from build123d import *

# Parameters (mm, degrees)
F4_D    = 6.4
F5_SIZE = 2


with BuildPart() as f1:
    # F0 (on Front) → F1 (revolve)
    with BuildSketch(Plane.XZ):
        Polygon((-44, 0), (-44, -2), (-2.715, -2), (-2.715, 10), (-60, 10), (-60, 0), align=None)
    revolve(axis=Axis((0, 0, 2.463164), (0, 0, -1)))

    # F4 (through all)
    with Locations(Plane.XY.offset(10)):
        with Locations((-26, 45.033321), (-52, 0), (-26, -45.033321), (26, -45.033321), (52, 0), (26, 45.033321)):
            Hole(F4_D / 2)

    # F5
    f5_edges = [f1.edges().sort_by_distance(p)[0] for p in [
        (60, 0, 10),
    ]]
    chamfer(f5_edges, length=F5_SIZE)

    # F6 (on Front) → F7 (revolve)
    with BuildSketch(Plane.XZ):
        with BuildLine():
            Line((-3.91, 45.97), (-3.91, 37.61))
            Line((-3.91, 37.61), (-5.085, 35.51))
            Line((-5.085, 35.51), (-5.085, 33.81))
            Line((-5.085, 33.81), (-3.91, 33.81))
            Line((-3.91, 33.81), (-3.91, 29.6))
            Line((-3.91, 29.6), (-5.09, 23.4))
            Line((-5.09, 23.4), (-5.09, 20.8))
            Line((-5.09, 20.8), (-3.91, 14.6))
            Line((-3.91, 14.6), (-6.95, 14.6))
            Line((-6.95, 14.6), (-6.95, 10))
            Line((-6.95, 10), (-2.715, 10))
            Line((-2.715, 10), (-2.715, 46.47))
            Line((-2.715, 46.47), (-3.41, 46.47))
            ThreePointArc((-3.41, 46.47), (-3.763553, 46.323553), (-3.91, 45.97))
        make_face()
    revolve(axis=Axis((0, 0, 24.371663), (0, 0, 1)))


solid = f1.part
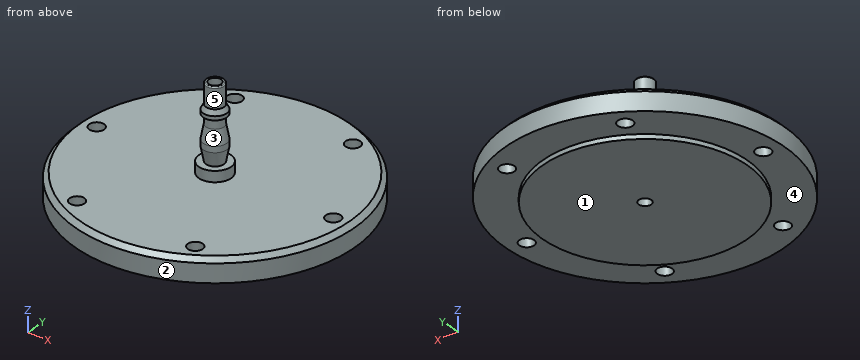
Here's how the part is built. I have some questions about the finished solid (model axes, mm). Face numbers are marked on the shaded views. A direction names the side the tool comes from. Round coordinates to 2 decimals unless told otherwise and drop trailing zeros. Write each loop counter-clockwise with the first axis right and the second up, starting at its lowest first coordinate (ties: lowest second). Pieces come first, ordered by that corner, then holes.
1. Suppose I cut it at B-B (y = 0). State how many separate pieces and enclosed holes the cut face has, and give its area (3 significant figures).
2. Suppose I cut it at D-D (z = 4.5). List the corners of the cut face in (x, y) for me (3 decimals).
3. I need wall thicknesses on L1, parallel to Y at x = 0, z = 38 (3 decimals); L2, parallel to Y at x = 0, z = 5.5 (3 decimals); L3, parallel to Y at x = -26, z = 7. Which ranges of each line are inside material? Lowest first, please.
4. If we mould it in two halves opening along Z, with no side actions, what happens to the marked faces 1, 2 and 3? For each: released by +Z, released by -Z, zero draft, split by the parting line, or undercut.
5. For the marked faces 4 and 5, which set-ups out of +Z, -Z, +X, -X, +Y, -Y let a thin tool reach every point of the face, with its end or its side?
6. Suppose I cut it at A-A (z = 12.5). List the corners of the cut face in (x, y) for me (3 decimals).
7. Will these pins go through, and if not, where does the flat tip stop? pin 1 Ø8.5 at (x, y) = (26, -45.03) entering from -Z; pin 2 Ø8.5 at (x, y) = (52, 0) entering from +Z; pin 3 Ø8 at (y, z) = (7.5, 4.5) entering from +X.
Answer sheet:
1. separate pieces: 4
1. enclosed holes: 0
1. area: 1,320 mm2
2. outline: circle Ø120 at (0, 0); hole circle Ø6.4 at (-52, 0); hole circle Ø6.4 at (-26, -45.033); hole circle Ø6.4 at (-26, 45.033); hole circle Ø5.43 at (0, 0); hole circle Ø6.4 at (26, -45.033); hole circle Ø6.4 at (26, 45.033); hole circle Ø6.4 at (52, 0)
3. L1: y = -3.91 to -2.715, 2.715 to 3.91
3. L2: y = -60 to -2.715, 2.715 to 60
3. L3: y = -54.07 to -48.23, -41.83 to 41.83, 48.23 to 54.07
4. face 1: released by -Z
4. face 2: zero draft
4. face 3: undercut
5. face 4: -Z
5. face 5: +Z
6. outline: circle Ø13.9 at (0, 0); hole circle Ø5.43 at (0, 0)
7. pin 1: stops at z = 0
7. pin 2: stops at z = 10
7. pin 3: stops at x = 59.9
